Check sheet for the modelled part. Datum: model origin and axes. Units: mm. A direction names the side the tool comes from. Round coordinates to 2 decimals unless told otherwise and drop trailing zeros. Loops run counter-clockwise (first coordinate to the right, second up) from the corner with the lowest first, then second, coordinate; pieces in that order, holes last. Notation, with made-up numbers: (-4, -16) -> (44, -16) arc R24 cw to (44, -3) -> close; hole circle Ø8 at (88, -21.5). An arc over 180 degrees is marked (long way). One line per item, written item: value. Start each with the question number.
1. Cross-section at D-D on x = 0. Record the cut outline in (y, z).
2. Cross-section at A-A on z = 0. Record the cut outline in (x, y), then the cut area to 3 significant figures.
3. Cross-section at B-B on x = 7.5. Record the cut outline in (y, z), then the cut area to 3 significant figures.
4. Release check for a two-part mould opening along Z. For faces 5 (the face through (0, 15, 0)), 6 (the face through (-9, 5, 2)), 7 (the face through (0, 13, -6)) record: +Z half, -Z half, draft (parallel to the pull), parting line (faces both ways), or undercut.
5. Set-up check for faces 1 (the face through (0.1, 10.2, -6.5)), 2 (the face through (-0.1, 10.2, 6.5)), 3 (the face through (-5.37, 2.46, -0.28)), 4 (the face through (3.595, 8.959, -0.867)): record each of +Z, -Z, +X, -X, +Y, -Y from which the full face is reachable in a straight line by a thin tool's end or side.
6. Material ranges on L1, parallel to X at y = 1.75, z = 0; L2, parallel to Y at x = 11.25, z = 1.5; L3, parallel to X at y = 12, z = 0, recorded low to high.
7. Cross-section at C-C on y = 8. Record the cut outline in (x, z), then the cut area to 3 significant figures.
8. Go/stop test with flat-tipped pins: pin 1 (1 mm diameter, centred on x = 7, y = 7.5, fed in from +Z); pin 2 (4 mm diameter, centred on x = 9.5, z = 1.5, fed in from +Y); pin 3 (2 mm diameter, centred on y = 13.5, z = 6.5, fed in from -X). Record where each tip stops, or that it passes through.
from build123d import *
from build123d.topology import SkipClean

# Parameters (mm, degrees)
SKETCH_1_R          = 12
SKETCH_1_R_2        = 2.15
EXTRUDE_1_DEPTH     = 15
CUT_EXTRUDE_START   = -5
SKETCH_2_R          = 12
CUT_EXTRUDE_1_DEPTH = 5
EXTRUDE_2_DEPTH     = 0.5
SKETCH_4_R          = 4
CUT_EXTRUDE_2_DEPTH = 10
FILLET_1_R          = 0.5


with BuildPart() as part:
    # ｽｹｯﾁ1 → ﾎﾞｽ - 押し出し1 (new body)
    with BuildSketch(Plane(origin=(0, 0, 0), x_dir=(1, 0, 0), z_dir=(0, 1, 0))):
        with Locations(Location((0, 0, 0), (0, 0, 270))):
            Circle(SKETCH_1_R)
        with Locations(Location((-7.5, 0, 0), (0, 0, 270))):
            Circle(SKETCH_1_R_2, mode=Mode.SUBTRACT)
        with Locations(Location((7.5, 0, 0), (0, 0, 90))):
            Circle(SKETCH_1_R_2, mode=Mode.SUBTRACT)
    extrude(amount=EXTRUDE_1_DEPTH)

    # ｽｹｯﾁ2 → ｶｯﾄ - 押し出し1 (cut)
    with BuildSketch(Plane(origin=(0, 15, 0), x_dir=(1, 0, 0), z_dir=(0, 1, 0)).offset(CUT_EXTRUDE_START)):
        with Locations(Location((0, 0, 0), (0, 0, 270))):
            Circle(SKETCH_2_R)
        with BuildLine():
            ThreePointArc((5.841833333, 1.368569803), (0, 6), (-5.841833333, 1.368569803))
            ThreePointArc((-5.841833333, 1.368569803), (-5.35, 0), (-5.841833333, -1.368569803))
            ThreePointArc((-5.841833333, -1.368569803), (0, -6), (5.841833333, -1.368569803))
            ThreePointArc((5.841833333, -1.368569803), (5.35, 0), (5.841833333, 1.368569803))
        make_face(mode=Mode.SUBTRACT)
    extrude(amount=CUT_EXTRUDE_1_DEPTH, mode=Mode.SUBTRACT)

    # ｽｹｯﾁ3 → ﾎﾞｽ - 押し出し2 (add)
    with SkipClean():  # the faces are left unmerged after this step: merging them gives an invalid solid
        with BuildSketch(Plane(origin=(0, 10, 0), x_dir=(1, 0, 0), z_dir=(0, 1, 0))):
            with BuildLine():
                ThreePointArc((-6.2585, -1.755328388), (0, -6.5), (6.2585, -1.755328388))
                ThreePointArc((6.2585, -1.755328388), (6.03732702, -1.575781633), (5.841833333, -1.368569803))
                ThreePointArc((5.841833333, -1.368569803), (5.35, 0), (5.841833333, 1.368569803))
                ThreePointArc((5.841833333, 1.368569803), (6.03732702, 1.575781633), (6.2585, 1.755328388))
                ThreePointArc((6.2585, 1.755328388), (0, 6.5), (-6.2585, 1.755328388))
                ThreePointArc((-6.2585, 1.755328388), (-6.03732702, 1.575781633), (-5.841833333, 1.368569803))
                ThreePointArc((-5.841833333, 1.368569803), (-5.35, 0), (-5.841833333, -1.368569803))
                ThreePointArc((-5.841833333, -1.368569803), (-6.03732702, -1.575781633), (-6.2585, -1.755328388))
            make_face()
        extrude(amount=EXTRUDE_2_DEPTH)

    # ｽｹｯﾁ4 → ｶｯﾄ - 押し出し2 (cut)
    with BuildSketch(Plane(origin=(0, 15, 0), x_dir=(1, 0, 0), z_dir=(0, 1, 0))):
        with Locations(Location((-7.5, 0, 0), (0, 0, 270))):
            Circle(SKETCH_4_R)
        with Locations(Location((7.5, 0, 0), (0, 0, 270))):
            Circle(SKETCH_4_R)
    extrude(amount=-CUT_EXTRUDE_2_DEPTH, mode=Mode.SUBTRACT)

    # ﾌｨﾚｯﾄ1
    fillet_1_edges = [part.edges().sort_by_distance(p)[0] for p in [
        (-5.083333333, 12.75, 3.187431916),
        (-5.083333333, 12.75, -3.187431916),
        (5.083333333, 12.75, 3.187431916),
        (5.083333333, 12.75, -3.187431916),
    ]]
    fillet(fillet_1_edges, radius=FILLET_1_R)


solid = part.part
Taken from the geometry:
1. outline: (0, -12) -> (10, -12) -> (10, -6.5) -> (10.5, -6.5) -> (10.5, -6) -> (15, -6) -> (15, 6) -> (10.5, 6) -> (10.5, 6.5) -> (10, 6.5) -> (10, 12) -> (0, 12) -> close
2. outline: (-12, 0) -> (-9.65, 0) -> (-9.65, 5) -> (-11.5, 5) -> (-11.5, 10) -> (-12, 10) -> close; (-5.35, 0) -> (5.35, 0) -> (5.35, 5) -> (3.5, 5) -> (3.5, 15) -> (-3.5, 15) -> (-3.5, 5) -> (-5.35, 5) -> close; (9.65, 0) -> (12, 0) -> (12, 10) -> (11.5, 10) -> (11.5, 5) -> (9.65, 5) -> close
2. area: 152 mm2
3. outline: (0, -9.37) -> (10, -9.37) -> (10, -4) -> (5, -4) -> (5, -2.15) -> (0, -2.15) -> close; (0, 2.15) -> (5, 2.15) -> (5, 4) -> (10, 4) -> (10, 9.37) -> (0, 9.37) -> close
3. area: 126 mm2
4. face 5: draft
4. face 6: undercut
4. face 7: -Z half
5. face 1: -Z, +Y
5. face 2: +Z, +Y
5. face 3: +Y, -Y
5. face 4: +Y
6. L1: x = -12 to -9.65, -5.35 to 5.35, 9.65 to 12
6. L2: y = 0 to 10
6. L3: x = -3.5 to 3.5
7. outline: circle Ø24 at (0, 0); hole circle Ø8 at (-7.5, 0); hole circle Ø8 at (7.5, 0)
7. area: 352 mm2
8. pin 1: stops at z = 10.09
8. pin 2: stops at y = 10
8. pin 3: stops at x = -2.4
